The listing builds one solid part. Answer for the finished solid, in the listing's coordinates (mm). Face numbers are marked on the shaded views. Round coordinates to 2 decimals unless told otherwise and drop trailing zeros. Write each loop counter-clockwise with the first axis right and the second up, starting at its lowest first coordinate (ties: lowest second). Pieces come first, ordered by that corner, then holes. Notation, with made-up numbers: M -34.5,-3 L -30.5,-3 A26 cw -30.5,25 Z; hole C 18.25,67.25 d4. An arc over 180 degrees is marked long. Put each result on its own line as item: value. Start each with the question number.
```python
from build123d import *

# Parameters (mm, degrees)
PAD_DEPTH            = 11
PAD_MIRRORED_2_DEPTH = 11


with BuildPart() as part:
    # Sketch → Pad (new body)
    with BuildSketch(Plane.XY):
        with BuildLine():
            Line((0, 0), (39, 0))
            ThreePointArc((51, 0), (45, 6), (39, 0))
            Line((51, 0), (55, 0))
            Line((55, 0), (55, 9))
            Line((55, 9), (0, 9))
            Line((0, 9), (0, 0))
        make_face()
    pad = extrude(amount=PAD_DEPTH)

    # Sketch Mirrored 2 → Pad Mirrored 2 (add)
    with BuildSketch(Plane(origin=(0, 0, 0), x_dir=(-1, 0, 0), z_dir=(0, 0, -1))):
        with BuildLine():
            Line((0, 0), (39, 0))
            ThreePointArc((51, 0), (45, 6), (39, 0))
            Line((51, 0), (55, 0))
            Line((55, 0), (55, 9))
            Line((55, 9), (0, 9))
            Line((0, 9), (0, 0))
        make_face()
    pad_mirrored_2 = extrude(amount=-PAD_MIRRORED_2_DEPTH)

    # Mirrored001: Pad, Pad Mirrored 2 across Sketch H_Axis
    add(pad.mirror(Plane.ZX))
    add(pad_mirrored_2.mirror(Plane.ZX))


solid = part.part
```
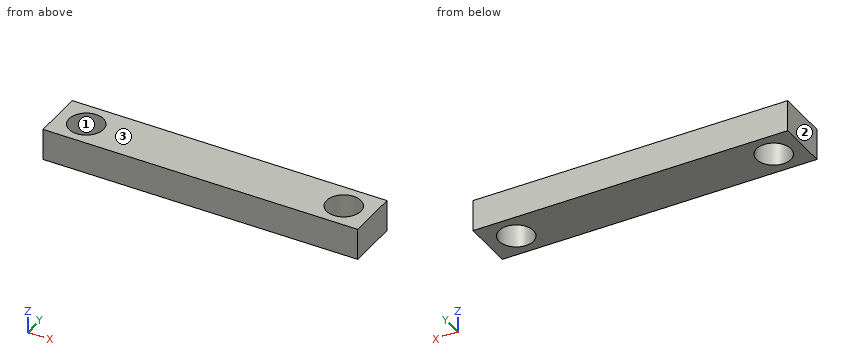
Item 1: Determine the mould class of the marked faces 1, 2 and 3 for opening direction X: released by +X, released by -X, zero draft, split by the parting line, or undercut.
Item 2: Consider line 1 along X through (y, z) = (0, 8); line 2 along Y through (x, z) = (45, 5); line 3 along X through (y, z) = (1.75, 9.25). Determine where each line is inside the solid, lowest interval first. Write a range as [from, to].
Item 3: Section C-C (z = 3) is taken. Give the vertices of the cut face in (x, y), and give its area (3 significant figures).
Item 4: Section A-A (x = -45) is taken. Give the vertices of the cut face in (y, z).
Item 5: Section B-B (y = 0) is taken. Give the vertices of the cut face in (x, z), and give its area (3 significant figures).
Output values:
1. face 1: undercut
1. face 2: released by -X
1. face 3: zero draft
2. line 1: x = [-55, -51], [-39, 39], [51, 55]
2. line 2: y = [-9, -6], [6, 9]
2. line 3: x = [-55, -50.74], [-39.26, 39.26], [50.74, 55]
3. outline: M -55,-9 L 55,-9 L 55,9 L -55,9 Z; hole C -45,0 d12; hole C 45,0 d12
3. area: 1,750 mm^2
4. outline: M -9,0 L -6,0 L -6,11 L -9,11 Z; M 6,0 L 9,0 L 9,11 L 6,11 Z
5. outline: M -55,0 L -51,0 L -51,11 L -55,11 Z; M -39,0 L 39,0 L 39,11 L -39,11 Z; M 51,0 L 55,0 L 55,11 L 51,11 Z
5. area: 946 mm^2
